Check sheet for the modelled part. Datum: model origin and axes. Units: mm. Face numbers are marked on the shaded views. A direction names the side the tool comes from. Give positions to 0.01 mm unless a question says otherwise; leave off trailing zeros. Loops run counter-clockwise (first coordinate to the right, second up) from the corner with the lowest first, then second, coordinate; pieces in that order, holes last. Notation, with made-up numbers: (66.5, -19.5) -> (100.5, -19.5) arc R21 ccw to (100.5, 6.5) -> close; hole circle Ø2 at (-25.5, 10.25). An arc over 180 degrees is marked (long way). Answer as CSV lines item,"result". Start each with the question number.
(1) Gauge pin test, flat ends, axial feed: pin 1 Ø8 at (x, z) = (35, 15) entering from +Y; pin 2 Ø12.5 at (x, z) = (20, 15) entering from -Y; pin 3 Ø4 at (y, z) = (27.5, 24) entering from -X; pin 4 Ø3 at (x, z) = (44, 15) entering from -Y. Record the tip position at first contact, or that the pin passes through.
(2) Section check B-B on x = 13. State how many separate pieces and enclosed holes the cut face has, plus the area to 3 significant figures.
(3) Access from +Z, -Z, +X, -X, +Y, -Y to the whole of each face (thin tool, end or side, straight path). Record for the marked faces 1, 2, 3, 4 and 5.
(4) Section check A-A on x = 24.5. Enter the section's corners in (y, z).
(5) Release check for a two-part mould opening along X. For the marked faces 6, 7 and 8 record: pulls with the +X half, pulls with the -X half, needs draft (parallel to the pull), parting line crosses it, or undercut.
(6) Section check D-D on y = 37. Enter the section's corners in (x, z).
(7) Material ranges on line 1 (Y direction, x = 15, z = 8.25); line 2 (Y direction, x = 9, z = 22); line 3 (X direction, y = 28, z = 15), recorded low to high. Write a range as from..to.
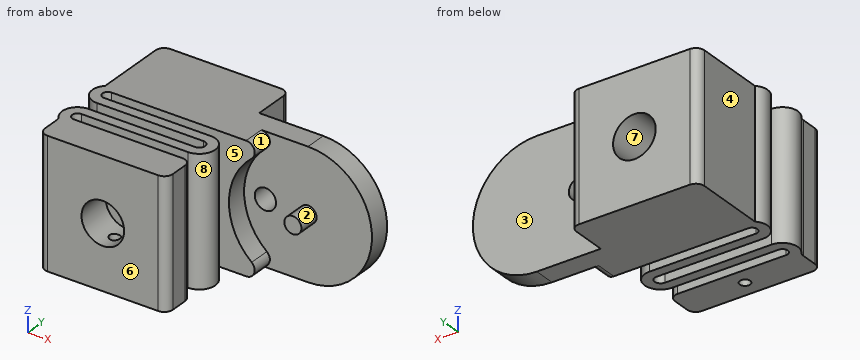
Autodesk Inventor part; units mm, degrees
ref_plane "YZ Plane" through (0, 0, 0) normal (1, 0, 0) x (0, 1, 0)
ref_plane "XZ Plane" through (0, 0, 0) normal (0, 1, 0) x (-1, 0, 0)
ref_plane "XY Plane" through (0, 0, 0) normal (0, 0, 1) x (1, 0, 0)
sketch "Skizze3" plane through (0, 0, 0) normal (0, 0, 1) x (1, 0, 0)
  line L0 (0, 0) -> (0, 8)
  line L1 (0, 8) -> (30, 8)
  line L2 (30, 0) -> (0, 0)
  arc A0 (2.5, 21.75) -> (2.5, 16.75) centre (2.5, 19.25) ccw construction
  arc A1 (27.5, 11.75) -> (27.5, 16.75) centre (27.5, 14.25) ccw construction
  line L3 (27.5, 16.75) -> (2.5, 16.75) construction
  line L4 (2.5, 11.75) -> (27.5, 11.75) construction
  arc A2 (2.5, 11.75) -> (0.3349, 8) centre (2.5, 9.25) ccw construction
  line L5 (0, 20.5) -> (0, 40.5)
  line L6 (0, 40.5) -> (30, 40.5)
  arc A3 (0, 21.8681) -> (2.5, 15.63) centre (2.5, 19.25) ccw
  line L7 (2.5, 15.63) -> (27.5, 15.63)
  arc A4 (27.5, 12.87) -> (27.5, 15.63) centre (27.5, 14.25) ccw
  line L8 (27.5, 12.87) -> (2.5, 12.87)
  arc A5 (2.5, 12.87) -> (0, 6.6319) centre (2.5, 9.25) ccw
  arc A6 (2.5, 20.5) -> (2.5, 18) centre (2.5, 19.25) ccw
  line L9 (2.5, 18) -> (27.5, 18)
  arc A7 (27.5, 10.5) -> (27.5, 18) centre (27.5, 14.25) ccw
  line L10 (27.5, 10.5) -> (2.5, 10.5)
  arc A8 (2.5, 10.5) -> (2.5, 8) centre (2.5, 9.25) ccw
  line L11 (0, 20.5) -> (30, 20.5)
  line L12 (30, 20.5) -> (30, 20.5)
  line L13 (30, 20.5) -> (30, 30.5)
  line L14 (30, 40.5) -> (30, 30.5)
  line L15 (30, 0) -> (30, 8)
  line L16 (30, 30.5) -> (60, 30.5)
  line L17 (60, 30.5) -> (60, 25.5)
  line L18 (30, 25.5) -> (60, 25.5)
  point P0 (15, 4)
  point P1 (0, 4)
  point P2 (15, 0)
  point P3 (30, 30.5)
  dimension "d4" = 8
  dimension "d11" = 5
  dimension "d12" = 5
  dimension "d17" = 5
  dimension "d19" = 1.12
  dimension "d20" = 1.25
  dimension "d22" = 20
  dimension "d23" = 30
  dimension "d54" = 30
  dimension "d71" = 5
  dimension "d72" = 5
  dimension "d73" = 30
extrude "Extrusion3" add sketch "Skizze3" along normal blind 30
sketch "Skizze4" plane through (30, 30.5, 0) normal (0, 1, 0) x (1, 0, 0)
  circle A0 centre (15, -15) radius 2
  circle A1 centre (5, -15) radius 2.5
  circle A2 centre (15, -15) radius 15
  line L0 (30, 0) -> (0, 0)
  line L1 (0, 0) -> (0, -30)
  line L2 (30, -30) -> (0, -30)
  line L3 (30, 0) -> (30, -30)
  circle A3 centre (15, -15) radius 15
  line L4 (0, 0) -> (0, -30)
  point P0 (0, -18)
  point P1 (25, -18)
  point P2 (24, -15)
  point P3 (29.5215, -11.2415)
  point P4 (-20, -18)
  point P5 (10.3125, -7.5196)
  point P6 (10.3125, -12.4804)
  point P7 (30, -15)
  point P8 (15, 0)
  point P9 (15, -30)
  point P10 (0, -15)
  point P11 (15, 0)
  point P12 (15, -30)
  dimension "d36" = 5
  dimension "d75" = 10
  dimension "d76" = 4
sketch "Skizze6" plane through (0, 40.5, 0) normal (0, 1, 0) x (1, 0, 0)
  circle A0 centre (15, -15) radius 5
  line L0 (30, -30) -> (0, -30)
  line L1 (0, 0) -> (0, -30)
  point P0 (15, -30)
  point P1 (0, -15)
  dimension "d51" = 10
extrude "Extrusion9" cut sketch "Skizze6" against normal through all
extrude "Extrusion6" cut sketch "Skizze4" against normal through all contours A1 | L3 L2 A2 | A2 L0 L3
extrude "Extrusion7" add sketch "Skizze4" against normal blind 10 contours A0 | A2 L1 L0 | L2 L1 A2
hole "Bohrung1" at (15, 4, 0) direction (0, 0, 1) diameter 2.459 end up to surface
fillet "Rundung3" radius 2 8 edges at (0, 40.5, 15) (30, 40.5, 15) (30, 0, 15) (30, 8, 15) (0, 0, 15) (0, 6.6319, 15) (45, 23, 0) (45, 23, 30)
equation "\"d12\" = d11"
properties part number "BT505_trajan20_22" material "Kunststoff, undurchsichtig Weiß"
Working result:
1,pin 1,"stops at y = 30.5"
1,pin 2,"stops at y = 0"
1,pin 3,"stops at x = 0"
1,pin 4,"stops at y = 20.5"
2,separate pieces,"8"
2,enclosed holes,"0"
2,area,"682 mm^2"
3,face 1,"+X, -Y"
3,face 2,"-Y"
3,face 3,"+Z, -Z, +X, +Y"
3,face 4,"+Z, -Z, -X, +Y"
3,face 5,"+Z, -Z, +X"
4,outline,"(0, 0) -> (8, 0) -> (8, 30) -> (0, 30) -> close; (10.5, 0) -> (12.87, 0) -> (12.87, 30) -> (10.5, 30) -> close; (15.63, 0) -> (18, 0) -> (18, 30) -> (15.63, 30) -> close; (20.5, 0) -> (40.5, 0) -> (40.5, 30) -> (20.5, 30) -> close"
5,face 6,"needs draft"
5,face 7,"undercut"
5,face 8,"pulls with the +X half"
6,outline,"(0, 0) -> (30, 0) -> (30, 30) -> (0, 30) -> close; hole circle Ø10 at (15, 15)"
7,line 1,"y = 0..2.77, 5.23..8, 10.5..12.87, 15.63..18, 20.5..40.5"
7,line 2,"y = 0..8, 10.5..12.87, 15.63..18, 20.5..40.5"
7,line 3,"x = 0..10, 20..32.5, 37.5..60"
